```python
from build123d import *


with BuildPart() as part:
    # Sketch1 → Revolve1 (revolve)
    with BuildSketch(Plane.XZ, mode=Mode.PRIVATE) as revolve1_sk:
        Polygon((6.5, 2.25), (6.25, 2.5), (5.25, 2.5), (5.25, 2), (2.75, 2), (2.75, 2.5), (1, 2.5), (1, -2.5), (2.75, -2.5), (2.75, -2), (5.25, -2), (5.25, -2.5), (6.25, -2.5), (6.5, -2.25), align=None)
    revolve(revolve1_sk.sketch.rotate(Axis((-1.5, 0, 2.5), (0, 0, -1)), 180), axis=Axis((-1.5, 0, 2.5), (0, 0, -1)))


solid = part.part
```
Input: part model. Units: mm. Frame: model coordinates. A direction names the side the tool comes from. Coordinates: 2 decimals unless noted, no trailing zeros. Loops run counter-clockwise (first coordinate to the right, second up) from the corner with the lowest first, then second, coordinate; pieces in that order, holes last. Notation, with made-up numbers: M 45,22.25 L 102,22.25 A22 cw 102,31.25 Z; hole C 26.5,50.5 d1. An arc over 180 degrees is marked long. Answer in a Markdown table with one row per item.
1. Draft query along X for faces 4 (the flat face through (-2, -3, -2.5)), 5 (the cylindrical face through (-5.19, -7.1, 0.03)), 6 (the cylindrical face through (-0.04, -6.59, 2.25)). Return one class per face: pulls with the +X half, pulls with the -X half, needs draft (parallel to the pull), parting line crosses it, or undercut.
Response:
| item | result |
|---|---|
| face 4 | needs draft |
| face 5 | parting line crosses it |
| face 6 | undercut |
2. Section B-B, the plane x = -1.5. Output: boundary loops of the cut face in (y, z).
Response:
| item | result |
|---|---|
| outline | M -8,-2.25 L -7.75,-2.5 L -6.75,-2.5 L -6.75,-2 L -4.25,-2 L -4.25,-2.5 L -2.5,-2.5 L -2.5,2.5 L -4.25,2.5 L -4.25,2 L -6.75,2 L -6.75,2.5 L -7.75,2.5 L -8,2.25 Z; M 2.5,-2.5 L 4.25,-2.5 L 4.25,-2 L 6.75,-2 L 6.75,-2.5 L 7.75,-2.5 L 8,-2.25 L 8,2.25 L 7.75,2.5 L 6.75,2.5 L 6.75,2 L 4.25,2 L 4.25,2.5 L 2.5,2.5 Z |
3. Section A-A, the plane y = 0. Output: boundary loops of the cut face in (x, z), then the cut area to 3 significant figures.
Response:
| item | result |
|---|---|
| outline | M -9.5,-2.25 L -9.25,-2.5 L -8.25,-2.5 L -8.25,-2 L -5.75,-2 L -5.75,-2.5 L -4,-2.5 L -4,2.5 L -5.75,2.5 L -5.75,2 L -8.25,2 L -8.25,2.5 L -9.25,2.5 L -9.5,2.25 Z; M 1,-2.5 L 2.75,-2.5 L 2.75,-2 L 5.25,-2 L 5.25,-2.5 L 6.25,-2.5 L 6.5,-2.25 L 6.5,2.25 L 6.25,2.5 L 5.25,2.5 L 5.25,2 L 2.75,2 L 2.75,2.5 L 1,2.5 Z |
| area | 49.9 mm2 |
4. First-contact query: pin 1 (1.5 mm diameter, centred on x = -6, z = -1, fed in from +Y). Flat tip, straight axial feed; report the tip coordinate or a pass-through.
Response:
| item | result |
|---|---|
| pin 1 | stops at y = 7.07 |
5. Section C-C, the plane z = -0.2. Output: boundary loops of the cut face in (x, y), then the cut area to 3 significant figures.
Response:
| item | result |
|---|---|
| outline | C -1.5,0 d16; hole C -1.5,0 d5 |
| area | 181 mm2 |
6. Material intervals for line 1 (Y direction, x = -1.5, z = 2.1); line 2 (Y direction, x = -1.5, z = -0.25); line 3 (Y direction, x = -2.5, z = -2.15), sorted ascending.
Response:
| item | result |
|---|---|
| line 1 | y = -8 to -6.75, -4.25 to -2.5, 2.5 to 4.25, 6.75 to 8 |
| line 2 | y = -8 to -2.5, 2.5 to 8 |
| line 3 | y = -7.94 to -6.68, -4.13 to -2.29, 2.29 to 4.13, 6.68 to 7.94 |
7. Reachability of faces 1 (the cylindrical face through (-0.947, 4.214, 2.254)), 2 (the flat face through (-1, 7, -2.5)), 3 (the flat face through (3, 0, -2)) from +Z, -Z, +X, -X, +Y, -Y: full face, straight path, thin tool, end or side. Return the list, or none.
Response:
| item | result |
|---|---|
| face 1 | +Z |
| face 2 | -Z, +X, -X, +Y, -Y |
| face 3 | -Z |
